Source: three-view drawing plus pictorial views. Frame: mm from the lowest corner of the part. Round coordinates to 2 decimals unless told otherwise and drop trailing zeros. Write each loop counter-clockwise with the first axis right and the second up, starting at its lowest first coordinate (ties: lowest second). Pieces come first, ordered by that corner, then holes. Notation, with made-up numbers: M 67.25,45.5 L 85.25,45.5 A26 ccw 85.25,62.5 Z; hole C 56.5,61 d1. An arc over 180 degrees is marked long. Put each result on its own line as item: value. Start each with the question number.
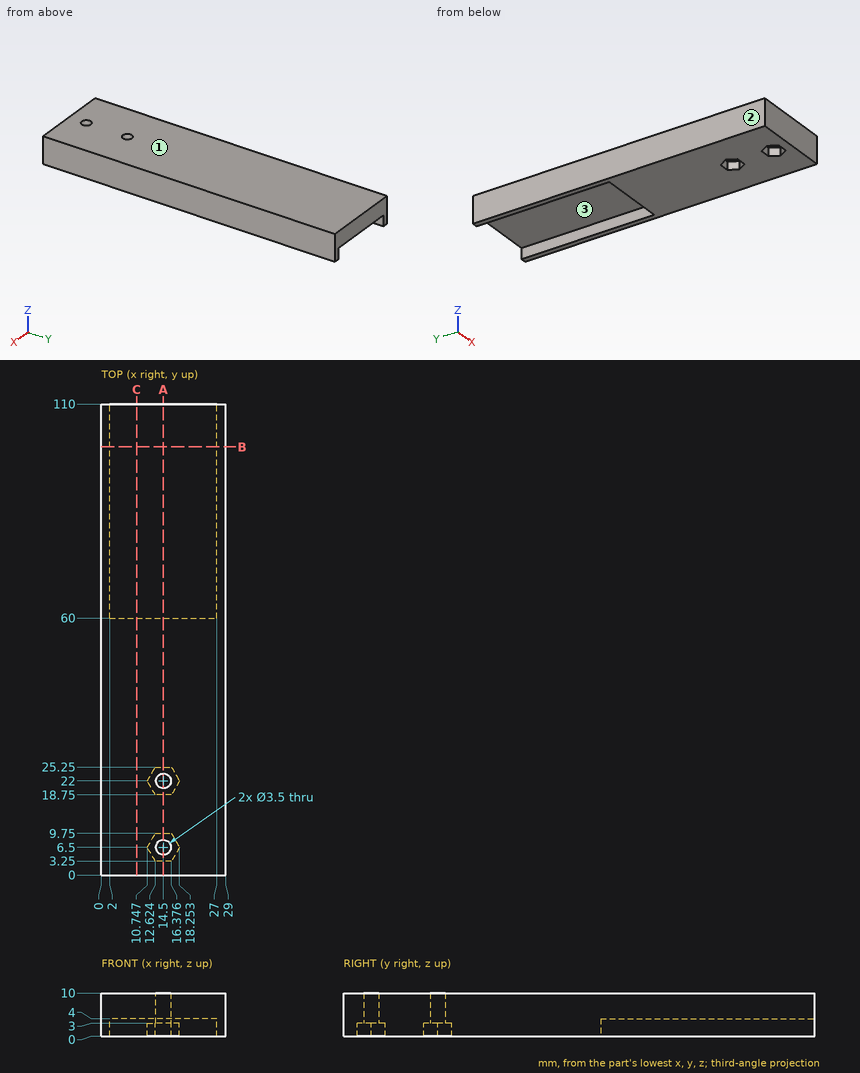
(1) Pull-direction query (X, two-part tool) for the marked faces 1, 2 and 3; classes: +X half, -X half, draft (parallel to the pull), parting line (faces both ways), or undercut.
(2) Contact query for flat-ended pins moving along their axis: P1, Ø0.9, axis at x = 14.5, z = 1.5, coming from the +Y side; P2, Ø2, axis at x = 14.5, y = 6.5, coming from the -Z side; P3, Ø7.5, axis at x = 15, y = 88.5, coming from the -Z side. Output: stop coordinate, or through.
(3) Section query A-A (x = 14.5). Return loops of the section in (y, z), and give its area (3 significant figures).
(4) Section query B-B (y = 100). Return loops of the section in (x, z), and give its area (3 significant figures).
(5) Section query C-C (x = 8.25). Return loops of the section in (y, z).
(6) Ray query, line 1 along Y through (x, z) = (14.5, 4.75); line 2 along Z through (x, y) = (20.5, 85); line 3 along Z through (x, y) = (13.5, 8). Return the intervals inside material, ascending.
Entries:
1. face 1: draft
1. face 2: -X half
1. face 3: undercut
2. P1: y = 60
2. P2: through
2. P3: z = 4
3. outline: M 0,0 L 3.25,0 L 3.25,3 L 4.75,3 L 4.75,10 L 0,10 Z; M 8.25,3 L 9.75,3 L 9.75,0 L 18.75,0 L 18.75,3 L 20.25,3 L 20.25,10 L 8.25,10 Z; M 23.75,3 L 25.25,3 L 25.25,0 L 60,0 L 60,4 L 110,4 L 110,10 L 23.75,10 Z
3. area: 812 mm2
4. outline: M 0,0 L 2,0 L 2,4 L 27,4 L 27,0 L 29,0 L 29,10 L 0,10 Z
4. area: 190 mm2
5. outline: M 0,0 L 60,0 L 60,4 L 110,4 L 110,10 L 0,10 Z
6. line 1: 0 to 4.75, 8.25 to 20.25, 23.75 to 110
6. line 2: 4 to 10
6. line 3: 3 to 10
